Design review of the part built by this model. Coordinates are the model's own, in mm. Give positions to 0.01 mm unless a question says otherwise; leave off trailing zeros. Write each loop counter-clockwise with the first axis right and the second up, starting at its lowest first coordinate (ties: lowest second). Pieces come first, ordered by that corner, then holes. Notation, with made-up numbers: (69.5, 47.25) - (122.5, 47.25) arc R14 ccw to (122.5, 64.25) - close; hole circle Ø1 at (-25.75, -18). An arc over 180 degrees is marked (long way). Write each question's results on one line, items separated by ' | '. Start each with the question number.
from build123d import *

# Parameters (mm, degrees)
SKETCH_1_R               = 4
SKETCH_1_R_2             = 3
EXTRUDE_1_DEPTH          = 230
CHAMFER_1_SIZE           = 0.3
CUT_EXTRUDE_1_DEPTH      = 231.0695547
CUT_EXTRUDE_1_DEPTH_BACK = 231.0695547
SKETCH_2_R               = 1


with BuildPart() as part:
    # Эскиз1 → Бобышка-Вытянуть1 (new body)
    with BuildSketch(Plane(origin=(0, 0, 0), x_dir=(1, 0, 0), z_dir=(0, 1, 0))):
        with Locations(Location((0, 0, 0), (0, 0, 270))):
            Circle(SKETCH_1_R)
        with Locations(Location((0, 0, 0), (0, 0, 270))):
            Circle(SKETCH_1_R_2, mode=Mode.SUBTRACT)
    extrude(amount=EXTRUDE_1_DEPTH)

    # Фаска1
    chamfer_1_edges = [part.edges().sort_by_distance(p)[0] for p in [
        (0, 0, -4),
        (0, 230, -4),
        (0, 0, -3),
        (0, 230, -3),
    ]]
    chamfer(chamfer_1_edges, length=CHAMFER_1_SIZE)

    # Эскиз2 → Вырез-Вытянуть1 (cut, two sides: drawn at the far end of the back side and taken through both)
    with BuildSketch(Plane(origin=(0, 0, 0), x_dir=(0, 0, -1), z_dir=(1, 0, 0)).offset(-CUT_EXTRUDE_1_DEPTH_BACK)):
        with Locations((0, 9)):
            Circle(SKETCH_2_R)
    extrude(amount=CUT_EXTRUDE_1_DEPTH + CUT_EXTRUDE_1_DEPTH_BACK, mode=Mode.SUBTRACT)


solid = part.part
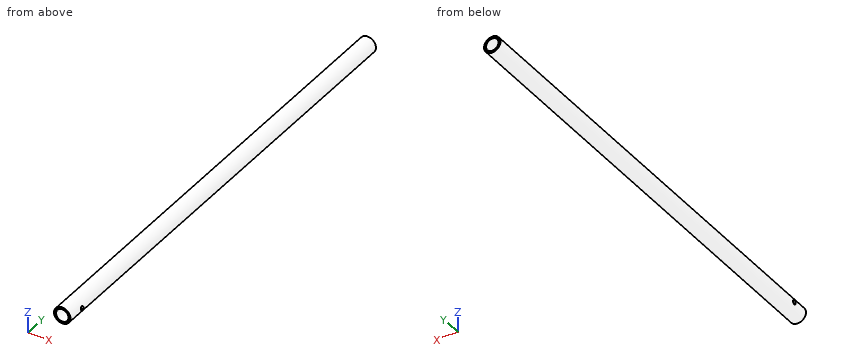
Q1. For line 1 along Y through (x, z) = (-3.35, 0); line 2 along X through (y, z) = (143, 0); line 3 along Z through (x, y) = (-0.75, 135.5), list the stretches that pass through material, from the lowest coordinate up. Write a range as [from, to].
Q2. Add section B-B on y = 74.5. State the section outline as (x, z) points, plus the area to 3 significant figures.
Q3. Insertion check: P1, Ø1, axis at x = 1.5, y = 167, coming from the +Z side; P2, Ø1.5, axis at x = -3, y = 147, coming from the -Z side. Each pin has a flat end and moves straight along its axis. Give the tip position at first contact, or say it passes through.
Q4. Add section A-A on x = 0. State the section outline as (y, z) points.
Result:
1) line 1: y = [0, 8], [10, 230] | line 2: x = [-4, -3], [3, 4] | line 3: z = [-3.93, -2.9], [2.9, 3.93]
2) outline: circle Ø8 at (0, 0); hole circle Ø6 at (0, 0) | area: 22.0 mm²
3) P1: stops at z = 3.87 | P2: stops at z = -3.31
4) outline: (0, -3.7) - (0.3, -4) - (229.7, -4) - (230, -3.7) - (230, -3.3) - (229.7, -3) - (0.3, -3) - (0, -3.3) - close; (0, 3.3) - (0.3, 3) - (229.7, 3) - (230, 3.3) - (230, 3.7) - (229.7, 4) - (0.3, 4) - (0, 3.7) - close
